Geometry: see drawing. Coordinates: mm, zero at the bounding-box minimum. Coordinates: 2 decimals unless noted, no trailing zeros. Write each loop counter-clockwise with the first axis right and the second up, starting at its lowest first coordinate (ties: lowest second). Pieces come first, ordered by that corner, then holes. Notation, with made-up numbers: (-12.5, 54.5) -> (8.5, 54.5) arc R28 cw to (8.5, 91.5) -> close; hole circle Ø8 at (50.25, 62). An arc over 180 degrees is marked (long way). Answer as a JSON object with one key per item and string values. Group by question number.
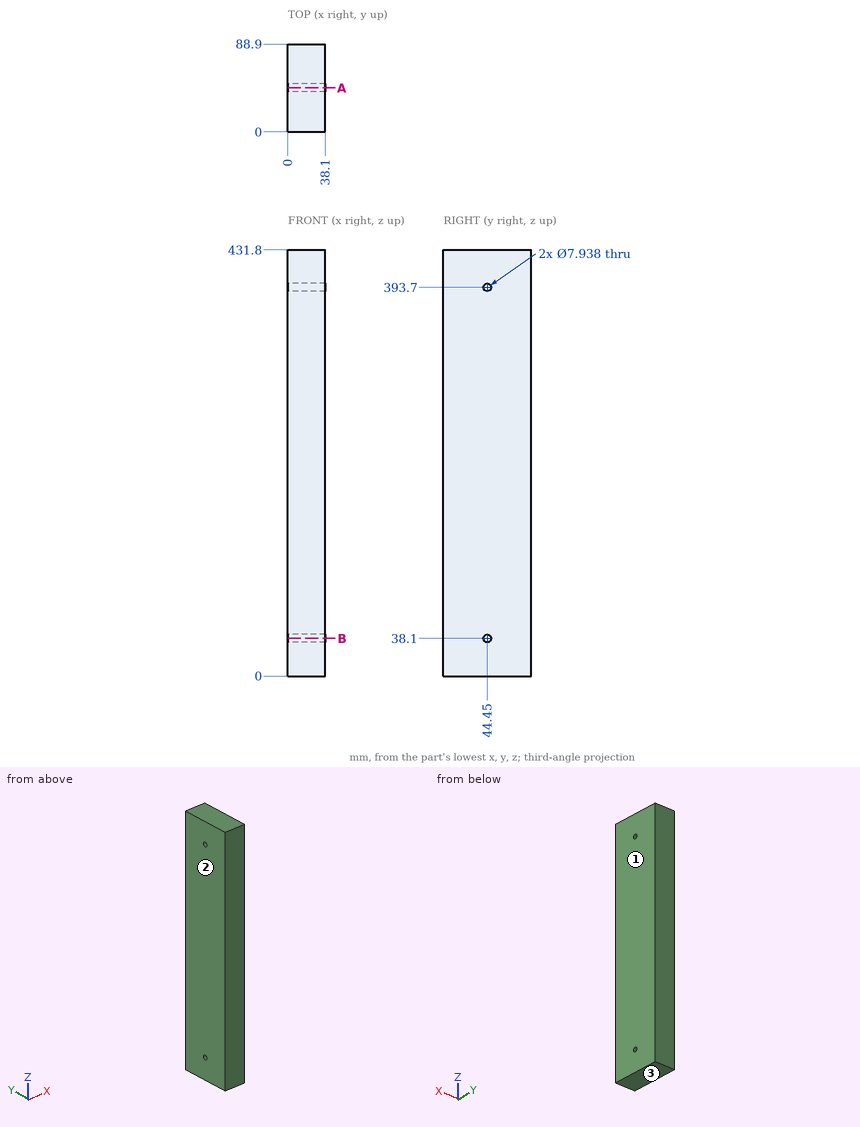
Item 1: Section A-A on y = 44.45. Output: boundary loops of the cut face in (x, z), then the cut area to 3 significant figures.
Item 2: Section B-B on z = 38.1. Output: boundary loops of the cut face in (x, y).
Item 3: Mould query, pull axis X, two halves, no side actions, for the marked faces 1, 2 and 3. Classes: +X half, -X half, draft (parallel to the pull), parting line (faces both ways), or undercut.
Item 4: Ray query, L1, parallel to Z at x = 20, y = 44; L2, parallel to Y at x = 11, z = 38; L3, parallel to Z at x = 13.5, y = 42. Return the intervals inside material, ascending. Write a range as [from, to].
Item 5: Contact query for a flat-ended pin moving along its axis: pin 1 (8 mm diameter, centred on x = 4, y = 40.5, fed in from -Z). Output: stop coordinate, or through.
Answer sheet:
{
 "1": {"outline": "(0, 0) -> (38.1, 0) -> (38.1, 34.13) -> (0, 34.13) -> close; (0, 42.07) -> (38.1, 42.07) -> (38.1, 389.73) -> (0, 389.73) -> close; (0, 397.67) -> (38.1, 397.67) -> (38.1, 431.8) -> (0, 431.8) -> close", "area": "15,800 mm^2"},
 "2": {"outline": "(0, 0) -> (38.1, 0) -> (38.1, 40.48) -> (0, 40.48) -> close; (0, 48.42) -> (38.1, 48.42) -> (38.1, 88.9) -> (0, 88.9) -> close"},
 "3": {"face 1": "+X half", "face 2": "-X half", "face 3": "draft"},
 "4": {"L1": "z = [0, 34.16], [42.04, 389.76], [397.64, 431.8]", "L2": "y = [0, 40.48], [48.42, 88.9]", "L3": "z = [0, 34.98], [41.22, 390.58], [396.82, 431.8]"},
 "5": {"pin 1": "stops at z = 0"}
}
